Can you work these out from the model? Positions are in its coordinate system, mm. A direction names the side the tool comes from. Coordinates: 2 decimals unless noted, no trailing zeros. Loops run counter-clockwise (first coordinate to the right, second up) from the corner with the lowest first, then second, coordinate; pieces in that order, holes last. Notation, with made-up numbers: M 77.5,37.5 L 95.5,37.5 A34 ccw 95.5,72.5 Z; hole C 66.5,-25 d8. An arc over 180 degrees is marked long. Answer as a JSON object with one key per item and string values. Group by question number.
Item 1: We'd pull the mould along Z, two halves only. Please class faces 1 (the cylindrical face through (185.074, 2.833, 149.019)), 2 (the flat face through (8.382, 3, 188)), 3 (the flat face through (169.518, 2.833, 172.854)): +Z half, -Z half, draft (parallel to the pull), parting line (faces both ways), or undercut.
Item 2: If I drill on line 1 (X direction, y = 0.45, z = 167.5); line 2 (X direction, y = 2, z = 164.5); line 3 (X direction, y = 2.1, z = 240.03), over which ranges is the centre line in solid material (lowest first)?
Item 3: Suppose I cut it at C-C (z = 226.5). Write out the boundary of the cut face in (x, y).
Item 4: Suppose I cut it at B-B (z = 89). Write out the boundary of the cut face in (x, y), then the cut area to 3 significant figures.
Item 5: Which directions (+Z, -Z, +X, -X, +Y, -Y) give clear straight access to the entire face, cutting with the end or side of a thin tool? Please do faces 4 (the cylindrical face through (153.6, 2.83, 76.73)), 5 (the flat face through (114.621, 2.833, 192.834)).
Item 6: I'm going to push a flat-ended pin straight in: pin 1 Ø1.5 at (y, z) = (3, 217.5) entering from +X. Where does the tip first touch, or does it pass through?
Item 7: Suppose I cut it at A-A (y = 4.35). Count the separate pieces of the cut face and the enclosed holes in it, then the cut area to 3 significant figures.
```python
from build123d import *

# Parameters (mm, degrees)
SKETCH1_R               = 7.366
SKETCH1_R_2             = 9.525
BOSS_EXTRUDE1_DEPTH     = 5.588
CUT_EXTRUDE1_DEPTH      = 334.830246753
CUT_EXTRUDE1_DEPTH_BACK = 334.830246753
SKETCH2_R               = 1.27
FILLET1_R               = 12.7
FILLET2_R               = 5.08
CUT_EXTRUDE3_DEPTH      = 334.830246753
CUT_EXTRUDE4_DEPTH      = 334.830246753
FILLET3_R               = 2.54
SKETCH6_R               = 1.27
CUT_EXTRUDE5_DEPTH      = 334.830246753


with BuildPart() as part:
    # Sketch1 → Boss-Extrude1 (new body)
    with BuildSketch(Plane(origin=(0, 0, 0), x_dir=(1, 0, 0), z_dir=(0, 1, 0))):
        with BuildLine():
            Line((8.382, -240.03), (8.382, -125.73))
            Line((8.382, -125.73), (155.947491633, -72.020553441))
            Line((155.947491633, -72.020553441), (184.566884059, -150.651687889))
            ThreePointArc((184.566884059, -150.651687889), (202.338954157, -156.340572379), (201.281045045, -174.970943032))
            ThreePointArc((201.281045045, -174.970943032), (129.350312262, -233.232473549), (41.837585925, -263.398))
            Line((41.837585925, -263.398), (31.75, -263.398))
            ThreePointArc((31.75, -263.398), (15.226328737, -256.553671263), (8.382, -240.03))
        make_face()
        with Locations(Location((31.75, -240.03, 0), (0, 0, 270))):
            Circle(SKETCH1_R, mode=Mode.SUBTRACT)
        with Locations(Location((189.779271043, -164.97260343, 0), (0, 0, 270))):
            Circle(SKETCH1_R_2, mode=Mode.SUBTRACT)
    extrude(amount=BOSS_EXTRUDE1_DEPTH)

    # Sketch2 → Cut-Extrude1 (cut, two sides: drawn at the far end of the back side and taken through both)
    with BuildSketch(Plane(origin=(0, 5.588, 0), x_dir=(1, 0, 0), z_dir=(0, 1, 0)).offset(-CUT_EXTRUDE1_DEPTH_BACK)):
        with Locations(Location((169.269931238, -179.701578394, 0), (0, 0, 270))):
            Circle(SKETCH2_R)
        with Locations(Location((119.146726846, -197.944932839, 0), (0, 0, 270))):
            Circle(SKETCH2_R)
        with Locations(Location((89.609867268, -116.793078108, 0), (0, 0, 270))):
            Circle(SKETCH2_R)
        with Locations(Location((139.733071661, -98.549723663, 0), (0, 0, 270))):
            Circle(SKETCH2_R)
    extrude(amount=CUT_EXTRUDE1_DEPTH + CUT_EXTRUDE1_DEPTH_BACK, mode=Mode.SUBTRACT)

    # Fillet1
    fillet1_edges = [part.edges().sort_by_distance(p)[0] for p in [
        (155.947491633, 2.794, 72.020553441),
        (8.382, 2.794, 125.73),
    ]]
    fillet(fillet1_edges, radius=FILLET1_R)

    # Fillet2
    fillet2_edges = [part.edges().sort_by_distance(p)[0] for p in [
        (184.566884059, 2.794, 150.651687889),
    ]]
    fillet(fillet2_edges, radius=FILLET2_R)

    # Sketch4 → Cut-Extrude3 (cut, through all)
    with BuildSketch(Plane(origin=(0, 5.588, 0), x_dir=(1, 0, 0), z_dir=(0, 1, 0))):
        with BuildLine():
            Line((95.57691541, -114.621250198), (93.839453082, -109.847611684))
            Line((93.839453082, -109.847611684), (132.028561191, -95.947913059))
            Line((132.028561191, -95.947913059), (133.766023519, -100.721551573))
            ThreePointArc((133.766023519, -100.721551573), (137.049445699, -104.304778111), (141.904899571, -104.516771805))
            Line((141.904899571, -104.516771805), (146.678538084, -102.779309477))
            Line((146.678538084, -102.779309477), (171.871741842, -171.997067924))
            Line((171.871741842, -171.997067924), (167.098103328, -173.734530252))
            ThreePointArc((167.098103328, -173.734530252), (163.514876791, -177.017952432), (163.302883096, -181.873406304))
            Line((163.302883096, -181.873406304), (165.040345424, -186.647044818))
            Line((165.040345424, -186.647044818), (126.851237316, -200.546743442))
            Line((126.851237316, -200.546743442), (125.113774988, -195.773104929))
            ThreePointArc((125.113774988, -195.773104929), (121.830352808, -192.189878391), (116.974898936, -191.977884697))
            Line((116.974898936, -191.977884697), (112.201260422, -193.715347025))
            Line((112.201260422, -193.715347025), (87.008056665, -124.497588578))
            Line((87.008056665, -124.497588578), (91.781695178, -122.76012625))
            ThreePointArc((91.781695178, -122.76012625), (95.364921716, -119.47670407), (95.57691541, -114.621250198))
        make_face()
    extrude(amount=-CUT_EXTRUDE3_DEPTH, mode=Mode.SUBTRACT)

    # Sketch5 → Cut-Extrude4 (cut, through all)
    with BuildSketch(Plane(origin=(0, 5.588, 0), x_dir=(1, 0, 0), z_dir=(0, 1, 0))):
        Polygon((110.680980885, -189.538413326), (89.199607574, -197.356993802), (84.855951753, -185.422897518), (106.337325065, -177.604317042), align=None)
    extrude(amount=-CUT_EXTRUDE4_DEPTH, mode=Mode.SUBTRACT)

    # Fillet3
    fillet3_edges = [part.edges().sort_by_distance(p)[0] for p in [
        (106.337325065, 2.794, 177.604317042),
        (110.680980885, 2.794, 189.538413326),
        (89.199607574, 2.794, 197.356993802),
        (84.855951753, 2.794, 185.422897518),
    ]]
    fillet(fillet3_edges, radius=FILLET3_R)

    # Sketch6 → Cut-Extrude5 (cut, through all)
    with BuildSketch(Plane(origin=(0, 5.588, 0), x_dir=(1, 0, 0), z_dir=(0, 1, 0))):
        with Locations(Location((51.420759159, -130.692776733, 0), (0, 0, 270))):
            Circle(SKETCH6_R)
        with Locations(Location((27.552566591, -139.380088373, 0), (0, 0, 270))):
            Circle(SKETCH6_R)
        with Locations(Location((48.402114528, -196.663750536, 0), (0, 0, 270))):
            Circle(SKETCH6_R)
        with Locations(Location((72.270307096, -187.976438896, 0), (0, 0, 270))):
            Circle(SKETCH6_R)
    extrude(amount=-CUT_EXTRUDE5_DEPTH, mode=Mode.SUBTRACT)


solid = part.part
```
From the geometry:
{
 "1": {"face 1": "-Z half", "face 2": "draft", "face 3": "undercut"},
 "2": {"line 1": "8.38 to 102.66, 170.23 to 180.6, 198.96 to 204.81", "line 2": "8.38 to 101.57, 169.14 to 180.27, 199.29 to 205.01", "line 3": "8.38 to 24.38, 39.12 to 116.25"},
 "3": {"outline": "M 8.38,0 L 140.81,0 L 140.81,5.59 L 8.38,5.59 Z"},
 "4": {"outline": "M 109.3,0 L 162.13,0 L 162.13,5.59 L 109.3,5.59 Z", "area": "295 mm2"},
 "5": {"face 4": "-Z, +Y, -Y", "face 5": "+Y, -Y"},
 "6": {"pin 1": "x = 155.4"},
 "7": {"separate pieces": "1", "enclosed holes": "11", "area": "18,900 mm2"}
}
